Autodesk Inventor part; units mm, degrees
ref_plane "YZ Plane" through (0, 0, 0) normal (1, 0, 0) x (0, 1, 0)
ref_plane "XZ Plane" through (0, 0, 0) normal (0, 1, 0) x (-1, 0, 0)
ref_plane "XY Plane" through (0, 0, 0) normal (0, 0, 1) x (1, 0, 0)
sketch "Sketch1" plane through (0, 0, 0) normal (0, 0, 1) x (1, 0, 0)
  line L0 (-750, 0) -> (750, 0) construction
  line L1 (750, 0) -> (750, -2100) construction
  line L2 (750, -2100) -> (110, -2700) construction
  line L3 (107.8152, -2700) -> (-107.8152, -2700)
  line L4 (-110, -2700) -> (-750, -2100) construction
  line L5 (-750, -2100) -> (-750, 0) construction
  arc A0 (745.2369, 0.4471) -> (-745.2369, 0.4471) centre (0, -7964.7662) ccw construction
  arc A1 (-750.6265, -4.7429) -> (-777.5832, -235) centre (7180.7944, -1050) ccw construction
  arc A2 (-777.5832, -235) -> (-750.1285, -2099.0286) centre (7180.7944, -1050) ccw construction
  arc A3 (750.1285, -2099.0286) -> (777.5832, -235) centre (-7180.7944, -1050) ccw construction
  arc A4 (777.5832, -235) -> (750.6265, -4.7429) centre (-7180.7944, -1050) ccw construction
  line L6 (-777.5832, -235) -> (777.5832, -235) construction
  arc A5 (-749.3229, -2100.7083) -> (-677.5699, -2174.8011) centre (5033.2984, 3427.5183) ccw construction
  line L7 (-750, -2100) -> (750, -2100) construction
  line L8 (-547.1729, -2035.7109) -> (-801.0834, -2306.5488) construction
  arc A6 (-677.5699, -2174.8011) -> (-111.6739, -2698.5946) centre (5033.2984, 3427.5183) ccw
  arc A7 (-745.2369, 0.4471) -> (-750.6265, -4.7429) centre (-744.6779, -5.5268) ccw construction
  arc A8 (750.6265, -4.7429) -> (745.2369, 0.4471) centre (744.6779, -5.5268) ccw construction
  arc A9 (-750.1285, -2099.0286) -> (-749.3229, -2100.7083) centre (-747.1545, -2098.6352) ccw construction
  arc A10 (111.6739, -2698.5946) -> (677.5699, -2174.8011) centre (-5033.2984, 3427.5183) ccw
  line L9 (553.8195, -2042.8006) -> (794.4368, -2299.4591) construction
  arc A11 (677.5699, -2174.8011) -> (749.3229, -2100.7083) centre (-5033.2984, 3427.5183) ccw construction
  arc A12 (749.3229, -2100.7083) -> (750.1285, -2099.0286) centre (747.1545, -2098.6352) ccw construction
  arc A13 (-111.6739, -2698.5946) -> (-107.8152, -2700) centre (-107.8152, -2694) ccw
  arc A14 (107.8152, -2700) -> (111.6739, -2698.5946) centre (107.8152, -2694) ccw
  point P0 (0, 0)
  point P1 (0, 0)
  point P2 (0, 0)
  point P3 (0, -2700)
  point P4 (-674.1281, -2171.1299)
  point P5 (674.1281, -2171.1299)
  dimension "d19" = 1500
  dimension "d20" = 2100
  dimension "d21" = 220
  dimension "d22" = 2700
  dimension "d23" = 8000
  dimension "d24" = 8000
  dimension "d25" = 8000
  dimension "d26" = 235
  dimension "d27" = 8000
  dimension "d28" = 104
  dimension "d29" = 6
  dimension "d30" = 3
  dimension "d31" = 8000
  dimension "d32" = 104
  dimension "d33" = 6
contour flange "Contour Flange1" sketch "Sketch1" thickness 3 bend radius 3 width 1000 along (0, 0, 1) mid plane no both sides no wall seen from (-400.9365, -2443.52, 0) lies toward (0.6792794, 0.7338798, 0) curves A6 A13 L3 A14 A10
bend "Bend1"
corner "Corner1"
equation "\"d19\" = Бак_ширина_общая"
equation "\"d20\" = Бак_высота_до_конуса"
equation "\"d21\" = Бак_брюхо_ширина_полки"
equation "\"d23\" = Бак_радиус_стенок_общий"
equation "\"d24\" = Бак_радиус_стенок_общий"
equation "\"d25\" = Бак_радиус_стенок_общий"
equation "\"d26\" = Бак_спина_длина_фланцев"
equation "\"d27\" = Бак_радиус_стенок_общий"
equation "\"d29\" = d41 + d42"
equation "\"d30\" = d41"
equation "\"d31\" = Бак_радиус_стенок_общий"
equation "\"d33\" = Thickness + BendRadius"
equation "\"d7\" = Thickness"
equation "\"d8\" = BendReliefWidth"
equation "\"d9\" = BendReliefDepth"
equation "\"d10\" = MinimumRemnant"
equation "\"d11\" = TransitionRadius"
equation "\"d13\" = BendRadius"
equation "\"d15\" = CornerReliefSize"
equation "\"d16\" = GapSize"
equation "\"d17\" = JacobiRadiusSize"
equation "\"BendRadius\" = Thickness"
equation "\"BendReliefWidth\" = Thickness"
equation "\"BendReliefDepth\" = 0.5 * Thickness"
equation "\"CornerReliefSize\" = 4 * Thickness"
equation "\"MinimumRemnant\" = 2 * Thickness"
equation "\"TransitionRadius\" = BendRadius"
equation "\"JacobiRadiusSize\" = BendRadius"
equation "\"GapSize\" = Thickness"
equation "\"d42\" = d41"
properties part number "МОО 030 лист брюхо 1" material "Stainless Steel"
Check sheet for the modelled part. Datum: model origin and axes. Units: mm. A direction names the side the tool comes from. Round coordinates to 2 decimals unless told otherwise and drop trailing zeros. Loops run counter-clockwise (first coordinate to the right, second up) from the corner with the lowest first, then second, coordinate; pieces in that order, holes last. Notation, with made-up numbers: (-28.5, 60.25) - (-14.5, 60.25) arc R20 cw to (-14.5, 70.25) - close; hole circle Ø2 at (1, -28.5). An arc over 180 degrees is marked (long way). Write item = value, one per line. Start each with the question number.
Q1. Depth check by flat-ended pin: P1, Ø6, axis at x = -505, z = 894, coming from the +Y side; P2, Ø12, axis at x = 515.5, z = 813.5, coming from the -Y side; P3, Ø8, axis at x = -313, z = 194.5, coming from the -Y side. Enter the tip coordinate at first touch or a pass-through.
Q2. Release check for a two-part mould opening along X. For faces 3 (the face through (402.86, -2437.65, 493)), 4 (the face through (404.9, -2439.85, 493)), 5 (the face through (2, -2700, 493)), 6 (the face through (-394.94, -2444.98, 493)) record: pulls with the +X half, pulls with the -X half, needs draft (parallel to the pull), parting line crosses it, or undercut.
Q3. Section check A-A (y = -2453). Record the boundary of the cut face in (x, z), plus the area to 3 significant figures.
Q4. Section check B-B (z = 240.5). Record the boundary of the cut face in (x, y), plus the area to 3 significant figures.
Q5. Thickness scan on L1, parallel to Y at x = 45, z = 211.5; L2, parallel to X at y = -2400.5, z = 382; L3, parallel to X at y = -2546, z = 704.5. Record the ranges inside material, lowest first.
Q6. Section check D-D (x = -68). Record the boundary of the cut face in (y, z).
Q7. Access from +Z, -Z, +X, -X, +Y, -Y to the whole of each face (thin tool, end or side, straight path). Record for faces 1 (the face through (2, -2697, 493)), 2 (the face through (-396.97, -2447.19, 493)).
Derived:
q1.P1 = -2338.42
q1.P2 = -2341.14
q1.P3 = -2527.3
q2.face_3 = undercut
q2.face_4 = pulls with the +X half
q2.face_5 = needs draft
q2.face_6 = undercut
q3.outline = (-390.68, 0) - (-386.25, 0) - (-386.25, 1000) - (-390.68, 1000) - close; (386.25, 0) - (390.68, 0) - (390.68, 1000) - (386.25, 1000) - close
q3.area = 8,850 mm^2
q4.outline = (-677.57, -2174.8) arc R8000 ccw to (-111.67, -2698.59) arc R6 ccw to (-107.82, -2700) - (107.82, -2700) arc R6 ccw to (111.67, -2698.59) arc R8000 ccw to (677.57, -2174.8) - (675.43, -2172.7) arc R7997 cw to (109.74, -2696.3) arc R3 cw to (107.82, -2697) - (-107.82, -2697) arc R3 cw to (-109.74, -2696.3) arc R7997 cw to (-675.43, -2172.7) - close
q4.area = 5,290 mm^2
q5.L1 = -2700 to -2697
q5.L2 = -447.05 to -442.67, 442.67 to 447.05
q5.L3 = -288.08 to -283.57, 283.57 to 288.08
q6.outline = (-2700, 0) - (-2697, 0) - (-2697, 1000) - (-2700, 1000) - close
q7.face_1 = +Z, -Z, +Y
q7.face_2 = +Z, -Z, -X, -Y
